Source: CAD feature listing. Evaluate the final solid. Frame: model axes, mm. Face numbers are marked on the shaded views. A direction names the side the tool comes from. Give positions to 0.01 mm unless a question says otherwise; leave off trailing zeros. Loops run counter-clockwise (first coordinate to the right, second up) from the corner with the lowest first, then second, coordinate; pieces in that order, holes last.
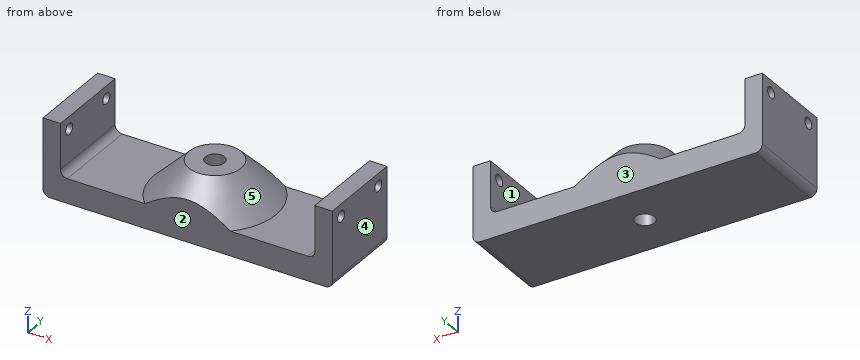
from build123d import *

# Parameters (mm, degrees)
SZKIC1_W                    = 83
SZKIC1_H                    = 25
DODANIE_WYCI_GNI_CIE1_DEPTH = 7
SZKIC2_W                    = 5
SZKIC2_H                    = 25
DODANIE_WYCI_GNI_CIE2_DEPTH = 15
WYTNIJ_WYCI_GNI_CIE1_REACH  = 88.771
SZKIC3_R                    = 1.6
SZKIC4_R                    = 7.5
DODANIE_WYCI_GNI_CIE4_DEPTH = 10
SZKIC5_R                    = 2.75
WYTNIJ_WYCI_GNI_CIE2_DEPTH  = 17
SFAZOWANIE1_SIZE            = 10
ZAOKR_GLENIE1_R             = 2
ZAOKR_GLENIE2_R             = 2


with BuildPart() as part:
    # Szkic1 → Dodanie-wyciągnięcie1 (new body)
    with BuildSketch(Plane.XY):
        Rectangle(SZKIC1_W, SZKIC1_H)
    extrude(amount=DODANIE_WYCI_GNI_CIE1_DEPTH)

    # Szkic2 → Dodanie-wyciągnięcie2 (add)
    with BuildSketch(Plane.XY.offset(7)):
        with Locations((-39, 0)):
            Rectangle(SZKIC2_W, SZKIC2_H)
        with Locations((39, 0)):
            Rectangle(SZKIC2_W, SZKIC2_H)
    extrude(amount=DODANIE_WYCI_GNI_CIE2_DEPTH)

    # Wytnij-wyciągnięcie1: up to this face of the body (flat: up to its plane)
    wytnij_wyci_gni_cie1_end = Plane(part.part.faces().sort_by_distance((-41.5, 0, 11))[0])
    # Szkic3 → Wytnij-wyciągnięcie1 (cut, up to the picked face)
    with BuildSketch(Plane(origin=(41.5, 0, 0), x_dir=(0, 0, -1), z_dir=(1, 0, 0)), mode=Mode.PRIVATE) as wytnij_wyci_gni_cie1_sk1:
        with Locations((-18.470012568, 8.5)):
            Circle(SZKIC3_R)
    wytnij_wyci_gni_cie1_tool1 = split(extrude(wytnij_wyci_gni_cie1_sk1.sketch, amount=-WYTNIJ_WYCI_GNI_CIE1_REACH, mode=Mode.PRIVATE), bisect_by=wytnij_wyci_gni_cie1_end, keep=Keep.BOTH, mode=Mode.PRIVATE)
    # Szkic3 → Wytnij-wyciągnięcie1 (cut, up to the picked face)
    with BuildSketch(Plane(origin=(41.5, 0, 0), x_dir=(0, 0, -1), z_dir=(1, 0, 0)), mode=Mode.PRIVATE) as wytnij_wyci_gni_cie1_sk2:
        with Locations((-18.470012568, -8.5)):
            Circle(SZKIC3_R)
    wytnij_wyci_gni_cie1_tool2 = split(extrude(wytnij_wyci_gni_cie1_sk2.sketch, amount=-WYTNIJ_WYCI_GNI_CIE1_REACH, mode=Mode.PRIVATE), bisect_by=wytnij_wyci_gni_cie1_end, keep=Keep.BOTH, mode=Mode.PRIVATE)
    add(wytnij_wyci_gni_cie1_tool1.solids().sort_by(Axis((41.5, 8.5, 18.470013), (-1, 0, 0)))[0], mode=Mode.SUBTRACT)
    add(wytnij_wyci_gni_cie1_tool2.solids().sort_by(Axis((41.5, -8.5, 18.470013), (-1, 0, 0)))[0], mode=Mode.SUBTRACT)

    # Szkic4 → Dodanie-wyciągnięcie4 (add)
    with BuildSketch(Plane.XY.offset(7)):
        with Locations(Location((0, 0, 0), (0, 0, 180))):
            Circle(SZKIC4_R)
    extrude(amount=DODANIE_WYCI_GNI_CIE4_DEPTH)

    # Szkic5 → Wytnij-wyciągnięcie2 (cut)
    with BuildSketch(Plane.XY.offset(17)):
        Circle(SZKIC5_R)
    extrude(amount=-WYTNIJ_WYCI_GNI_CIE2_DEPTH, mode=Mode.SUBTRACT)

    # Sfazowanie1
    # the kernel refuses this chamfer: 10 mm, written as the material it adds along each edge
    with BuildSketch(Plane(origin=(0, 0, 7), x_dir=(-1, 0, 0), z_dir=(0, 1, 0))) as sfazowanie1_piece_1_section:
        Polygon((7.5 + SFAZOWANIE1_SIZE, 0), (7.5, SFAZOWANIE1_SIZE), (7.5, 0), align=None)
    sfazowanie1_piece_1 = revolve(axis=Axis((0, 0, 7), (0, 0, 1)), mode=Mode.PRIVATE)
    sfazowanie1_piece_1 = split(sfazowanie1_piece_1, bisect_by=Plane(origin=(12.53571583, 12.5, 11.752873117), z_dir=(0, -1, 0)), keep=Keep.TOP, mode=Mode.PRIVATE)
    sfazowanie1_piece_1 = split(sfazowanie1_piece_1, bisect_by=Plane(origin=(12.53571583, -12.5, 11.752873117), z_dir=(0, 1, 0)), keep=Keep.TOP, mode=Mode.PRIVATE)
    sfazowanie1_piece_1 = split(sfazowanie1_piece_1, bisect_by=Plane(origin=(12.53571583, 0, 17), z_dir=(0, 0, -1)), keep=Keep.TOP, mode=Mode.PRIVATE)
    add(sfazowanie1_piece_1)

    # Zaokrąglenie1
    zaokr_glenie1_edges = [part.edges().sort_by_distance(p)[0] for p in [
        (-36.5, 0, 7),
        (36.5, 0, 7),
    ]]
    fillet(zaokr_glenie1_edges, radius=ZAOKR_GLENIE1_R)

    # Zaokrąglenie2
    zaokr_glenie2_edges = [part.edges().sort_by_distance(p)[0] for p in [
        (41.5, 0, 0),
        (-41.5, 0, 0),
    ]]
    fillet(zaokr_glenie2_edges, radius=ZAOKR_GLENIE2_R)


solid = part.part
1) Cut plane D-D (x = 19). Return loops of the section in (y, z), and give its area (3 significant figures).
Checks:
outline: (-12.5, 0) - (12.5, 0) - (12.5, 7) - (-12.5, 7) - close
area: 175 mm2
2) Contact query for flat-ended pins moving along their axis: P1, Ø2, axis at x = 8, z = 13.5, coming from the -Y side; P2, Ø6, axis at x = -0.5, y = -8.5, coming from the +Z side; P3, Ø6.5, axis at x = -28, y = 0, coming from the +Z side; P4, Ø4.5, axis at x = 0, y = 0, coming from the +Z side. Output: stop coordinate, or through.
Checks:
P1: stops at y = -9.2
P2: stops at z = 17
P3: stops at z = 7
P4: passes through
3) Reachability of the marked faces 1 and 2 from +Z, -Z, +X, -X, +Y, -Y: full face, straight path, thin tool, end or side. Return the list, or none.
Checks:
face 1: +Z, +Y, -Y
face 2: +Z, -Z, +X, -X, -Y
4) Cut plane B-B (y = 0). Return loops of the section in (x, z).
Checks:
outline: (-41.5, 2) arc R2 ccw to (-39.5, 0) - (-2.75, 0) - (-2.75, 17) - (-7.5, 17) - (-17.5, 7) - (-34.5, 7) arc R2 cw to (-36.5, 9) - (-36.5, 22) - (-41.5, 22) - close; (2.75, 0) - (39.5, 0) arc R2 ccw to (41.5, 2) - (41.5, 22) - (36.5, 22) - (36.5, 9) arc R2 cw to (34.5, 7) - (17.5, 7) - (7.5, 17) - (2.75, 17) - close
5) Pull-direction query (X, two-part tool) for the marked faces 3, 4 and 5; classes: released by +X, released by -X, zero draft, split by the parting line, or undercut.
Checks:
face 3: zero draft
face 4: released by +X
face 5: undercut
6) Cut plane A-A (x = 0). Return loops of the section in (y, z), and give its area (4 significant figures).
Checks:
outline: (-12.5, 0) - (-2.75, 0) - (-2.75, 17) - (-7.5, 17) - (-12.5, 12) - close; (2.75, 0) - (12.5, 0) - (12.5, 12) - (7.5, 17) - (2.75, 17) - close
area: 306.5 mm2
7) Cut plane C-C (z = 18). Return loops of the section in (x, y), and give its area (3 significant figures).
Checks:
outline: (-41.5, -12.5) - (-36.5, -12.5) - (-36.5, -10.03) - (-41.5, -10.03) - close; (-41.5, -6.97) - (-36.5, -6.97) - (-36.5, 6.97) - (-41.5, 6.97) - close; (-41.5, 10.03) - (-36.5, 10.03) - (-36.5, 12.5) - (-41.5, 12.5) - close; (36.5, -12.5) - (41.5, -12.5) - (41.5, -10.03) - (36.5, -10.03) - close; (36.5, -6.97) - (41.5, -6.97) - (41.5, 6.97) - (36.5, 6.97) - close; (36.5, 10.03) - (41.5, 10.03) - (41.5, 12.5) - (36.5, 12.5) - close
area: 189 mm2
8) Ray query, probe 1 along X at (y, z) = (5.25, 17.75); probe 2 along X at (y, z) = (-1.5, 7.5); probe 3 along X at (y, z) = (1.75, 12.25). Return the intervals inside material, ascending.
Checks:
probe 1: x = -41.5 to -36.5, 36.5 to 41.5
probe 2: x = -41.5 to -35.82, -16.93 to -2.3, 2.3 to 16.93, 35.82 to 41.5
probe 3: x = -41.5 to -36.5, -12.12 to -2.12, 2.12 to 12.12, 36.5 to 41.5
